Read the model definition and answer for the solid it produces. Units are mm, in the model's axes. A direction names the side the tool comes from. Coordinates: 2 decimals unless noted, no trailing zeros. Order: outer loops, then holes, each group sorted by start corner. A loop starts at its lowest first (then second) coordinate and runs counter-clockwise, first axis right, second up. Notation, with made-up numbers: M -6,27 L 26,27 A26 cw 26,60 Z; hole C 58.25,53 d10. An arc over 180 degrees is marked long. One line per question, with ' | ' between items. Start each with the question number.
1) Find section A-A, the plane y = -142. Write down the section's boundary in (x, z).
2) The mould has two halves that part along Y. Classify faces 4 (the face through (-129, -163, -4)), 5 (the face through (-199, -30, 6)), 6 (the face through (-200, -94, 6)): +Y half, -Y half, draft (parallel to the pull), parting line (faces both ways), or undercut.
3) Find section D-D, the plane z = 2. Count the separate pieces of the cut face and the enclosed holes in it, plus the area to 3 significant figures.
4) Given P1, Ø1, axis at y = -85, z = 10, coming from the +X side; P2, Ø3, axis at x = -84.5, z = 5.5, coming from the +Y side, each flat-ended and moving along its own axis, determine where each tip first touches the part or whether it passes through.
5) Consider probe 1 along Y at (x, z) = (-212.5, 3.5); probe 2 along X at (y, z) = (-162.5, 8.5); probe 3 along Y at (x, z) = (-185.5, 3.75). Determine where each line is inside the solid, lowest interval first.
6) Find section B-B, the plane y = -162.5. Write down the section's boundary in (x, z), plus the area to 3 significant figures.
7) A tool of negligible diameter and unlimited length cuts with its end or side. For faces 1 (the face through (-125.45, -108.18, 5.92)), 2 (the face through (-225, -104, 6)), 3 (the face through (-149, -85, 0)), from which of +Z, -Z, +X, -X, +Y, -Y can it reach the whole face along a straight path? Write none if from no direction.
8) Find section C-C, the plane x = -212.5. Write down the section's boundary in (y, z).
from build123d import *

# Parameters (mm, degrees)
F1_DEPTH  = 12
F2_W      = 200
F2_H      = 20
F3_DEPTH  = 5
F4_W      = 155
F4_H      = 20
F5_DEPTH  = 5
F6_R      = 2.5
F7_DEPTH  = 25
F9_DEPTH  = 5
F10_W     = 195
F10_H     = 30
F10_W_2   = 30
F10_H_2   = 145
F11_DEPTH = 25
F12_W     = 145
F12_H     = 9
F13_DEPTH = 195.0010001
F15_DEPTH = 25
F17_DEPTH = 25


with BuildPart() as f1:
    # F0 (on Top) → F1 (new body)
    with BuildSketch(Plane.XY):
        with BuildLine():
            add(Edge.make_bspline(
                [(-176, 0), (-176, -130), (0, -130)],
                knots=[3.1415926536, 3.1415926536, 3.1415926536, 4.7123889804, 4.7123889804, 4.7123889804], degree=2, weights=[1, 0.7071067812, 1]))
            Line((-176, 0), (-176, -130))
            Line((-176, -130), (0, -130))
        make_face()
        Polygon((-176, -130), (-176, 0), (-200, 0), (-200, -150), (0, -150), (0, -130), align=None)
    extrude(amount=F1_DEPTH)

    # F2 (on face) → F3 (join)
    with BuildSketch(Plane.XZ.offset(150)):
        with Locations((-100, 6)):
            Rectangle(F2_W, F2_H)
    extrude(amount=F3_DEPTH)

    # F4 (on face) → F5 (join)
    with BuildSketch(Plane(origin=(-200, 0, 0), x_dir=(0, -1, 0), z_dir=(-1, 0, 0))):
        with Locations((77.5, 6)):
            Rectangle(F4_W, F4_H)
    extrude(amount=F5_DEPTH)

    # F6 (on face) → F7 (join)
    with BuildSketch(Plane(origin=(0, 0, -4), x_dir=(1, 0, 0), z_dir=(0, 0, -1))):
        Polygon((0, 155), (0, 175), (-225, 175), (-225, 0), (-205, 0), (-205, 155), align=None)
        with Locations((-212.5, 60)):
            Circle(F6_R, mode=Mode.SUBTRACT)
        with Locations((-212.5, 115)):
            Circle(F6_R, mode=Mode.SUBTRACT)
        with Locations((-165, 162.5)):
            Circle(F6_R, mode=Mode.SUBTRACT)
        with Locations((-60, 162.5)):
            Circle(F6_R, mode=Mode.SUBTRACT)
    extrude(amount=-F7_DEPTH)

    # F8 (on face) → F9 (join)
    with BuildSketch(Plane.XY.offset(16)):
        Polygon((-190, 0), (-205, 0), (-205, -155), (0, -155), (0, -140), (-190, -140), align=None)
    extrude(amount=F9_DEPTH)

    # F10 (on Top) → F11 (cut, symmetric)
    with BuildSketch(Plane.XY):
        with Locations((-127.5, -15)):
            Rectangle(F10_W, F10_H)
        with Locations((-15, -15)):
            Rectangle(F10_W_2, F10_H)
        with Locations((-15, -102.5)):
            Rectangle(F10_W_2, F10_H_2)
    extrude(amount=F11_DEPTH, both=True, mode=Mode.SUBTRACT)

    # F12 (on face) → F13 (cut, through all)
    with BuildSketch(Plane.YZ.offset(-30)):
        with Locations((-102.5, 16.5)):
            Rectangle(F12_W, F12_H)
    extrude(amount=-F13_DEPTH, mode=Mode.SUBTRACT)

    # F14 (on face) → F15 (cut)
    with BuildSketch(Plane(origin=(0, 0, 0), x_dir=(1, 0, 0), z_dir=(0, 0, -1))):
        with BuildLine():
            ThreePointArc((-181.2494979045, 40), (-124.4154289012, 108.9058025162), (-40, 138.0975202339))
            Line((-40, 138.0975202339), (-40, 150))
            Line((-40, 150), (-200, 150))
            Line((-200, 150), (-200, 40))
            Line((-200, 40), (-181.2494979045, 40))
        make_face()
    extrude(amount=-F15_DEPTH, mode=Mode.SUBTRACT)

    # F16 (on face) → F17 (cut, through all)
    with BuildSketch(Plane.YZ.offset(-200)):
        Polygon((-150, 0), (-150, -4), (-30, -4), (-30, 0), (-40, 0), align=None)
    extrude(amount=-F17_DEPTH, mode=Mode.SUBTRACT)


solid = f1.part
Report:
1) outline: M -225,0 L -200,0 L -200,12 L -225,12 Z; M -40,0 L -30,0 L -30,12 L -40,12 Z
2) face 4: draft | face 5: +Y half | face 6: undercut
3) separate pieces: 1 | enclosed holes: 5 | area: 10,600 mm^2
4) P1: stops at x = -132.58 | P2: stops at y = -113.42
5) probe 1: y = -175 to -117.5, -112.5 to -62.5, -57.5 to -30 | probe 2: x = -225 to -167.5, -162.5 to -62.5, -57.5 to -30 | probe 3: y = -175 to -150, -40 to -30
6) outline: M -225,-4 L -167.5,-4 L -167.5,12 L -225,12 Z; M -162.5,-4 L -62.5,-4 L -62.5,12 L -162.5,12 Z; M -57.5,-4 L -30,-4 L -30,12 L -57.5,12 Z | area: 2,960 mm^2
7) face 1: +Z, -Z | face 2: +Z, -Z, -X, +Y, -Y | face 3: -Z, +X, -X, +Y
8) outline: M -175,-4 L -150,-4 L -150,0 L -117.5,0 L -117.5,12 L -175,12 Z; M -112.5,0 L -62.5,0 L -62.5,12 L -112.5,12 Z; M -57.5,0 L -30,0 L -30,12 L -57.5,12 Z
